from build123d import *

# Parameters (mm, degrees)
EXTRUDE1_DEPTH         = 6
EXTRUDE2_DEPTH         = 6
PROCESS_BENDS1_START   = 42.277322868
PROCESS_BENDS1_DEPTH   = 6
PROCESS_BENDS1_START_2 = -147.75
PROCESS_BENDS1_2_DEPTH = 295.5
PROCESS_BENDS1_START_3 = -135.25
PROCESS_BENDS1_3_DEPTH = 270.5
PROCESS_BENDS1_START_4 = -145.75
PROCESS_BENDS1_4_DEPTH = 291.5
PROCESS_BENDS1_5_DEPTH = 6


with BuildPart() as part:
    # Sketch1 → Extrude1 (new body)
    with BuildSketch(Plane.XY):
        with BuildLine():
            Line((-135.25, 0), (135.25, 0))
            ThreePointArc((135.25, 0), (136.591640787, 0.316718427), (137.65, 1.2))
            Line((137.65, 1.2), (145.15, 11.2))
            ThreePointArc((145.15, 11.2), (145.596049894, 12.051316702), (145.75, 13))
            Line((145.75, 13), (145.75, 2290))
            Line((145.75, 2290), (135.75, 2305))
            Line((135.75, 2305), (13, 2305))
            ThreePointArc((13, 2305), (10.878679656, 2304.121320344), (10, 2302))
            Line((10, 2302), (10, 2300))
            ThreePointArc((10, 2300), (0, 2290), (-10, 2300))
            Line((-10, 2300), (-10, 2302))
            ThreePointArc((-10, 2302), (-10.878679656, 2304.121320344), (-13, 2305))
            Line((-13, 2305), (-135.75, 2305))
            Line((-135.75, 2305), (-145.75, 2290))
            Line((-145.75, 2290), (-145.75, 13))
            ThreePointArc((-145.75, 13), (-145.596049894, 12.051316702), (-145.15, 11.2))
            Line((-145.15, 11.2), (-137.65, 1.2))
            ThreePointArc((-137.65, 1.2), (-136.591640787, 0.316718427), (-135.25, 0))
        make_face()
    extrude(amount=EXTRUDE1_DEPTH)

    # Sketch3 → Extrude2 (add)
    with BuildSketch(Plane.XY.offset(6)):
        with BuildLine():
            Line((147.348076211, 2142.232050808), (146.151923789, 2144.303847577))
            ThreePointArc((146.151923789, 2144.303847577), (145.852222521, 2145.027390442), (145.75, 2145.803847577))
            Line((145.75, 2145.803847577), (145.75, 2129.196152423))
            ThreePointArc((145.75, 2129.196152423), (145.852222521, 2129.972609558), (146.151923789, 2130.696152423))
            Line((146.151923789, 2130.696152423), (147.348076211, 2132.767949192))
            ThreePointArc((147.348076211, 2132.767949192), (147.647777479, 2133.491492057), (147.75, 2134.267949192))
            Line((147.75, 2134.267949192), (147.75, 2140.732050808))
            ThreePointArc((147.75, 2140.732050808), (147.647777479, 2141.508507943), (147.348076211, 2142.232050808))
        make_face()
        with BuildLine():
            Line((-145.75, 2129.196152423), (-145.75, 2145.803847577))
            ThreePointArc((-145.75, 2145.803847577), (-145.852222521, 2145.027390442), (-146.151923789, 2144.303847577))
            Line((-146.151923789, 2144.303847577), (-147.348076211, 2142.232050808))
            ThreePointArc((-147.348076211, 2142.232050808), (-147.647777479, 2141.508507943), (-147.75, 2140.732050808))
            Line((-147.75, 2140.732050808), (-147.75, 2134.267949192))
            ThreePointArc((-147.75, 2134.267949192), (-147.647777479, 2133.491492057), (-147.348076211, 2132.767949192))
            Line((-147.348076211, 2132.767949192), (-146.151923789, 2130.696152423))
            ThreePointArc((-146.151923789, 2130.696152423), (-145.852222521, 2129.972609558), (-145.75, 2129.196152423))
        make_face()
        with BuildLine():
            Line((145.75, 149.196152423), (145.75, 165.803847577))
            ThreePointArc((145.75, 165.803847577), (145.852222521, 165.027390442), (146.151923789, 164.303847577))
            Line((146.151923789, 164.303847577), (147.348076211, 162.232050808))
            ThreePointArc((147.348076211, 162.232050808), (147.647777479, 161.508507943), (147.75, 160.732050808))
            Line((147.75, 160.732050808), (147.75, 154.267949192))
            ThreePointArc((147.75, 154.267949192), (147.647777479, 153.491492057), (147.348076211, 152.767949192))
            Line((147.348076211, 152.767949192), (146.151923789, 150.696152423))
            ThreePointArc((146.151923789, 150.696152423), (145.852222521, 149.972609558), (145.75, 149.196152423))
        make_face()
        with BuildLine():
            Line((-147.348076211, 162.232050808), (-146.151923789, 164.303847577))
            ThreePointArc((-146.151923789, 164.303847577), (-145.852222521, 165.027390442), (-145.75, 165.803847577))
            Line((-145.75, 165.803847577), (-145.75, 149.196152423))
            ThreePointArc((-145.75, 149.196152423), (-145.852222521, 149.972609558), (-146.151923789, 150.696152423))
            Line((-146.151923789, 150.696152423), (-147.348076211, 152.767949192))
            ThreePointArc((-147.348076211, 152.767949192), (-147.647777479, 153.491492057), (-147.75, 154.267949192))
            Line((-147.75, 154.267949192), (-147.75, 160.732050808))
            ThreePointArc((-147.75, 160.732050808), (-147.647777479, 161.508507943), (-147.348076211, 162.232050808))
        make_face()
    extrude(amount=-EXTRUDE2_DEPTH)

    # Process-Bends1 2 outline → Process-Bends1 2 (cut)
    with BuildSketch(Plane.YZ.offset(PROCESS_BENDS1_START_2)):
        Polygon((92.396611983, 0), (80.736895303, 6), (0, 6), (0, 0), align=None)
        with BuildLine():
            Line((770.847206555, 6), (93.849827585, 6))
            Line((93.849827585, 6), (105.509544266, 0))
            Line((105.509544266, 0), (689.517739901, 0))
            Line((689.517739901, 0), (768.911335172, 5.927830646))
            ThreePointArc((768.911335172, 5.927830646), (769.878598478, 5.981951397), (770.847206555, 6))
        make_face()
    extrude(amount=PROCESS_BENDS1_2_DEPTH, mode=Mode.SUBTRACT)

    # Process-Bends1 3 outline → Process-Bends1 3 (add)
    with BuildSketch(Plane.YZ.offset(PROCESS_BENDS1_START_3)):
        Polygon((22.221302391, 42.859484921), (19.475921021, 37.524423428), (80.736895303, 6), (93.849827585, 6), align=None)
        with BuildLine():
            Line((105.509544266, 0), (92.396611983, 0))
            Line((92.396611983, 0), (171.747570561, -40.833389396))
            ThreePointArc((171.747570561, -40.833389396), (178.469550701, -43.194639768), (185.580094549, -43.64262024))
            Line((185.580094549, -43.64262024), (769.358074722, -0.055514888))
            ThreePointArc((769.358074722, -0.055514888), (770.102123419, -0.013883541), (770.847206555, 0))
            Line((770.847206555, 0), (689.517739901, 0))
            Line((689.517739901, 0), (185.133354999, -37.659274706))
            ThreePointArc((185.133354999, -37.659274706), (179.663705885, -37.314674343), (174.492951931, -35.498327904))
            Line((174.492951931, -35.498327904), (105.509544266, 0))
        make_face()
    extrude(amount=PROCESS_BENDS1_3_DEPTH)



with BuildPart() as body_2:
    # Process-Bends1: read off the stored shape, not the designer's step
    # Process-Bends1 outline → Process-Bends1 (new body)
    with BuildSketch(Plane(origin=(0, 0, 0), x_dir=(1, 0, 0), z_dir=(0, 0.457563561703474, 0.889176915468025)).offset(PROCESS_BENDS1_START)):
        with BuildLine():
            ThreePointArc((-145.75, 165.951578122), (-145.852222521, 165.175120987), (-146.151923789, 164.451578122))
            Line((-146.151923789, 164.451578122), (-147.348076211, 162.379781352))
            ThreePointArc((-147.348076211, 162.379781352), (-147.647777479, 161.656238487), (-147.75, 160.879781352))
            Line((-147.75, 160.879781352), (-147.75, 154.415679737))
            ThreePointArc((-147.75, 154.415679737), (-147.647777479, 153.639222602), (-147.348076211, 152.915679737))
            Line((-147.348076211, 152.915679737), (-146.151923789, 150.843882967))
            ThreePointArc((-146.151923789, 150.843882967), (-145.852222521, 150.120340102), (-145.75, 149.343882967))
            Line((-145.75, 149.343882967), (-145.75, 165.951578122))
        make_face()
        with BuildLine():
            Line((145.75, 165.951578122), (145.75, 149.343882967))
            ThreePointArc((145.75, 149.343882967), (145.852222521, 150.120340102), (146.151923789, 150.843882967))
            Line((146.151923789, 150.843882967), (147.348076211, 152.915679737))
            ThreePointArc((147.348076211, 152.915679737), (147.647777479, 153.639222602), (147.75, 154.415679737))
            Line((147.75, 154.415679737), (147.75, 160.879781352))
            ThreePointArc((147.75, 160.879781352), (147.647777479, 161.656238487), (147.348076211, 162.379781352))
            Line((147.348076211, 162.379781352), (146.151923789, 164.451578122))
            ThreePointArc((146.151923789, 164.451578122), (145.852222521, 165.175120987), (145.75, 165.951578122))
        make_face()
    extrude(amount=PROCESS_BENDS1_DEPTH)


with BuildPart() as part_1:
    add(part.part)

    add(body_2.part)  # Process-Bends1 4 merges body 2
    # Process-Bends1 4 outline → Process-Bends1 4 (add)
    with BuildSketch(Plane.YZ.offset(PROCESS_BENDS1_START_4)):
        with BuildLine():
            Line((105.509544266, 0), (92.396611983, 0))
            Line((92.396611983, 0), (171.747570561, -40.833389396))
            ThreePointArc((171.747570561, -40.833389396), (178.469550701, -43.194639768), (185.580094549, -43.64262024))
            Line((185.580094549, -43.64262024), (769.358074722, -0.055514888))
            ThreePointArc((769.358074722, -0.055514888), (770.102123419, -0.013883541), (770.847206555, 0))
            Line((770.847206555, 0), (689.517739901, 0))
            Line((689.517739901, 0), (185.133354999, -37.659274706))
            ThreePointArc((185.133354999, -37.659274706), (179.663705885, -37.314674343), (174.492951931, -35.498327904))
            Line((174.492951931, -35.498327904), (105.509544266, 0))
        make_face()
    extrude(amount=PROCESS_BENDS1_4_DEPTH)

    # Process-Bends1 5 outline → Process-Bends1 5 (add)
    with BuildSketch(Plane(origin=(0, 0, 0), x_dir=(1, 0, 0), z_dir=(0, 0.457563561703474, 0.889176915468025)).offset(PROCESS_BENDS1_START)):
        with BuildLine():
            Line((-145.75, 82), (-145.75, 13.147730544))
            ThreePointArc((-145.75, 13.147730544), (-145.596049894, 12.199047246), (-145.15, 11.347730544))
            Line((-145.15, 11.347730544), (-137.65, 1.347730544))
            ThreePointArc((-137.65, 1.347730544), (-136.591640786, 0.464448971), (-135.25, 0.147730544))
            Line((-135.25, 0.147730544), (-135.25, 82))
            Line((-135.25, 82), (-145.75, 82))
        make_face()
        with BuildLine():
            Line((145.75, 82), (135.25, 82))
            Line((135.25, 82), (135.25, 0.147730544))
            ThreePointArc((135.25, 0.147730544), (136.591640786, 0.464448971), (137.65, 1.347730544))
            Line((137.65, 1.347730544), (145.15, 11.347730544))
            ThreePointArc((145.15, 11.347730544), (145.596049894, 12.199047246), (145.75, 13.147730544))
            Line((145.75, 13.147730544), (145.75, 82))
        make_face()
    extrude(amount=PROCESS_BENDS1_5_DEPTH)


solid = part_1.part
Model file for the job. Use its own axes, mm. A direction names the side the tool comes from. Give positions to 0.01 mm unless a question says otherwise; leave off trailing zeros. Loops run counter-clockwise (first coordinate to the right, second up) from the corner with the lowest first, then second, coordinate; pieces in that order, holes last. Notation, with made-up numbers: (71.25, 15.25) - (104.25, 15.25) arc R19 ccw to (104.25, 28.25) - close; hole circle Ø11 at (18, 45). An arc over 180 degrees is marked (long way). Use one line per item in the form item = value.
(1) Cut at C-C (y = 724). Give the cut face in (x, z), then the cut area to 3 significant figures.
Determined:
outline = (-145.75, -3.44) - (145.75, -3.44) - (145.75, 2.57) - (-145.75, 2.57) - close
area = 1,750 mm^2
(2) Cut at B-B (y = 1384). Give the cut face in (x, z), then the cut area to 3 significant figures.
Determined:
outline = (-145.75, 0) - (145.75, 0) - (145.75, 6) - (-145.75, 6) - close
area = 1,750 mm^2
(3) Cut at A-A (x = -89.5). Give the cut face in (y, z), then the cut area to 3 significant figures.
Determined:
outline = (19.48, 37.52) - (171.75, -40.83) arc R26 ccw to (185.58, -43.64) - (769.36, -0.06) arc R20 cw to (770.85, 0) - (2305, 0) - (2305, 6) - (770.85, 6) arc R26 ccw to (768.91, 5.93) - (185.13, -37.66) arc R20 cw to (174.49, -35.5) - (22.22, 42.86) - close
area = 13,800 mm^2
(4) Drill centre lines: L1, parallel to Z at x = 35, y = 807; L2, parallel to Z at x = 55, y = 163.5; L3, parallel to Y at x = 13, z = 9.5. Where is each one in solid material? Low to high.
Determined:
L1 = 0 to 6
L2 = -36.59 to -29.84
L3 = 73.94 to 87.05
(5) Drop flat-ended pins along their axis: P1, Ø5, axis at y = 2201.5, z = 3.5, coming from the -X side; P2, Ø1.6, axis at y = 2301, z = 3.5, coming from the +X side; P3, Ø12, axis at x = 27.5, y = 1217, coming from the -Z side. Give the stop position or say it passes through.
Determined:
P1 = -145.75
P2 = 138.95
P3 = 0
(6) 3-axis set-ups, long thin cutter, end or side, ignore diameter. For faces 1 (the face through (-2, 1549, 6)), 2 (the face through (-145.75, 93, 3)), 3 (the face through (-2.04, 481.11, -15.56)), 4 (the face through (-2, 1549, 0)): which of +Z, -Z, +X, -X, +Y, -Y reach the whole face in a straight line?
Determined:
face_1 = +Z, +X, -X, +Y
face_2 = +Z, -Z, -X, -Y
face_3 = +Z, +X, -X
face_4 = -Z, +X, -X, +Y
